from build123d import *

# Parameters (mm, degrees)
SKETCH1_W               = 359.9
SKETCH1_H               = 87.2
BOSS_EXTRUDE1_DEPTH     = 1.6256
SKETCH2_W               = 359.9
SKETCH2_H               = 87.2
SKETCH2_W_2             = 356.6488
SKETCH2_H_2             = 83.9488
BOSS_EXTRUDE2_DEPTH     = 69.85
SKETCH3_W               = 416.6488
SKETCH3_H               = 138
SKETCH3_W_2             = 356.6488
SKETCH3_H_2             = 83.9488
BOSS_EXTRUDE3_DEPTH     = 1.6256
FILLET1_R               = 1.905
SKETCH6_W               = 371.0088
SKETCH6_H               = 92.8388
BOSS_EXTRUDE4_DEPTH     = 3.175
SKETCH8_R               = 7.62
CUT_EXTRUDE2_DEPTH      = 402.075797246
CUT_EXTRUDE4_DEPTH      = 232.308973187
CUT_EXTRUDE4_DEPTH_BACK = 232.308973187
SKETCH17_W              = 28.095
SKETCH17_H              = 54
CUT_EXTRUDE5_DEPTH      = 232.308973187
CUT_EXTRUDE5_DEPTH_BACK = 232.308973187
SKETCH18_R              = 3.325


with BuildPart() as part:
    # Sketch1 → Boss-Extrude1 (new body)
    with BuildSketch(Plane(origin=(0, 0, 0), x_dir=(1, 0, 0), z_dir=(0, 1, 0))):
        Rectangle(SKETCH1_W, SKETCH1_H)
    extrude(amount=BOSS_EXTRUDE1_DEPTH)

    # Sketch2 → Boss-Extrude2 (add)
    with BuildSketch(Plane(origin=(0, 1.6256, 0), x_dir=(1, 0, 0), z_dir=(0, 1, 0))):
        Rectangle(SKETCH2_W, SKETCH2_H)
        Rectangle(SKETCH2_W_2, SKETCH2_H_2, mode=Mode.SUBTRACT)
    extrude(amount=BOSS_EXTRUDE2_DEPTH)

    # Sketch3 → Boss-Extrude3 (add)
    with BuildSketch(Plane(origin=(0, 71.4756, 0), x_dir=(1, 0, 0), z_dir=(0, 1, 0))):
        Rectangle(SKETCH3_W, SKETCH3_H)
        Rectangle(SKETCH3_W_2, SKETCH3_H_2, mode=Mode.SUBTRACT)
    extrude(amount=BOSS_EXTRUDE3_DEPTH)

    # Fillet1
    fillet1_edges = [part.edges().sort_by_distance(p)[0] for p in [
        (0, 71.4756, -43.6),
        (-179.95, 71.4756, 0),
        (0, 71.4756, 43.6),
        (179.95, 71.4756, 0),
        (-178.3244, 73.1012, 0),
        (0, 73.1012, 41.9744),
        (178.3244, 73.1012, 0),
        (0, 73.1012, -41.9744),
    ]]
    fillet(fillet1_edges, radius=FILLET1_R)

    # Sketch6 → Boss-Extrude4 (add)
    with BuildSketch(Plane(origin=(0, 73.1012, 0), x_dir=(1, 0, 0), z_dir=(0, 1, 0))):
        Polygon((188.2394, -49.5944), (-188.2394, -49.5944), (-191.4144, -49.5944), (-191.4144, 49.5944), (-188.2394, 49.5944), (188.2394, 49.5944), (191.4144, 49.5944), (191.4144, -49.5944), align=None)
        with Locations((-2.735, 0)):
            Rectangle(SKETCH6_W, SKETCH6_H, mode=Mode.SUBTRACT)
    extrude(amount=-BOSS_EXTRUDE4_DEPTH)

    # Sketch8 → Cut-Extrude2 (cut, through all)
    with BuildSketch(Plane(origin=(179.95, 0, 0), x_dir=(0, 0, -1), z_dir=(1, 0, 0))):
        with Locations((0, 12.7)):
            Circle(SKETCH8_R)
    extrude(amount=-CUT_EXTRUDE2_DEPTH, mode=Mode.SUBTRACT)

    # Sketch17 → Cut-Extrude4 (cut, two sides: drawn at the far end of the back side and taken through both)
    with BuildSketch(Plane(origin=(0, 73.1012, 0), x_dir=(1, 0, 0), z_dir=(0, 1, 0)).offset(-CUT_EXTRUDE4_DEPTH_BACK)):
        with Locations((194.2769, 0)):
            Rectangle(SKETCH17_W, SKETCH17_H)
    extrude(amount=CUT_EXTRUDE4_DEPTH + CUT_EXTRUDE4_DEPTH_BACK, mode=Mode.SUBTRACT)

    # Sketch18 → Cut-Extrude5 (cut, two sides: drawn at the far end of the back side and taken through both)
    with BuildSketch(Plane(origin=(0, 73.1012, 0), x_dir=(1, 0, 0), z_dir=(0, 1, 0)).offset(-CUT_EXTRUDE5_DEPTH_BACK)):
        with Locations(Location((203.37295269, 41.64816795, 0), (0, 0, 270))):
            Circle(SKETCH18_R)
        with Locations(Location((203.37295269, -41.64816795, 0), (0, 0, 90))):
            Circle(SKETCH18_R)
        with Locations(Location((129.76878637, 57.22406113, 0), (0, 0, 270))):
            Circle(SKETCH18_R)
        with Locations(Location((-50.23121363, 57.22406113, 0), (0, 0, 270))):
            Circle(SKETCH18_R)
        with Locations(Location((39.76878637, 57.22406113, 0), (0, 0, 270))):
            Circle(SKETCH18_R)
        with Locations(Location((-140.23121363, 57.22406113, 0), (0, 0, 270))):
            Circle(SKETCH18_R)
        with Locations(Location((129.76878637, -57.22406113, 0), (0, 0, 90))):
            Circle(SKETCH18_R)
        with Locations(Location((39.76878637, -57.22406113, 0), (0, 0, 90))):
            Circle(SKETCH18_R)
        with Locations(Location((-50.23121363, -57.22406113, 0), (0, 0, 90))):
            Circle(SKETCH18_R)
        with Locations(Location((-140.23121363, -57.22406113, 0), (0, 0, 90))):
            Circle(SKETCH18_R)
    extrude(amount=CUT_EXTRUDE5_DEPTH + CUT_EXTRUDE5_DEPTH_BACK, mode=Mode.SUBTRACT)


solid = part.part
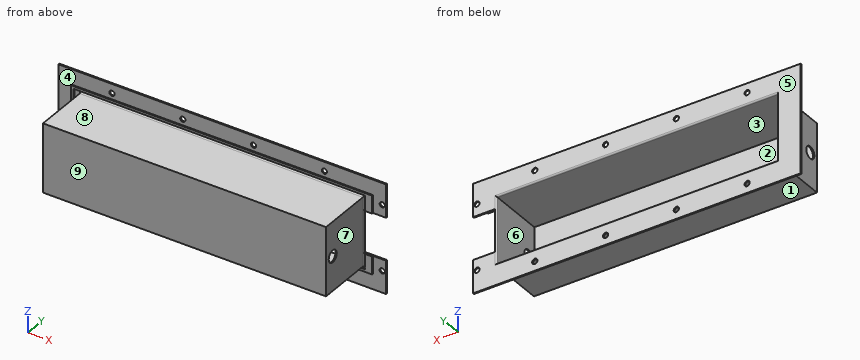
Can you work these out from the model? Positions are in its coordinate system, mm. Face numbers are marked on the shaded views. A direction names the side the tool comes from. Give positions to 0.01 mm unless a question says otherwise; leave off trailing zeros. Order: outer loops, then holes, each group sorted by start corner. A loop starts at its lowest first (then second) coordinate and runs counter-clockwise, first axis right, second up. Notation, with made-up numbers: M 58,18.5 L 67,18.5 A26 ccw 67,39.5 Z; hole C 31.25,68.25 d5. An arc over 180 degrees is marked long. Use a Markdown table: item, result. Add a question column.
Item 1: Suppose I cut it at B-B (y = 12.7). List the corners of the cut face in (x, z) for me, then the cut area to 3 significant figures.
Item 2: For the marked faces 5, 6, 7, 8 and 9, which set-ups out of +Z, -Z, +X, -X, +Y, -Y let a thin tool reach every point of the face, with its end or its side?
Item 3: Suppose I cut it at A-A (z = 0). List the corners of the cut face in (x, y) for me (3 decimals).
Item 4: We'd pull the mould along Z, two halves only. Please class the marked faces 1, 2, 3 and 4: +Z half, -Z half, draft (parallel to the pull), parting line (faces both ways), or undercut.
Item 5: Suppose I cut it at C-C (y = 52.5). List the corners of the cut face in (x, z) for me, then the cut area to 3 significant figures.
Item 6: If I drill on L1, parallel to Z at x = 88, y = 53.5; L2, parallel to X at y = 38, z = 18; L3, parallel to Z at x = -179, y = 12, over which ranges is the centre line in solid material (lowest first)? Write a range as [from, to].
Item 7: Suppose I cut it at D-D (x = -58). List the corners of the cut face in (y, z) for me (3 decimals).
Item 8: Will these pins go through, and if not, where does the flat tip stop? pin 1 (0.5 mm diameter, centred on y = 70.5, z = 38.5, fed in from -X); pin 2 (8 mm diameter, centred on y = 54.5, z = 31.5, fed in from -X); pin 3 (7.5 mm diameter, centred on x = -50.23, z = -57.22, fed in from -Y).
Answer sheet:
| question | item | result |
|---|---|---|
| 1 | outline | M -179.95,-43.6 L 179.95,-43.6 L 179.95,-7.62 L 178.32,-7.62 L 178.32,-41.97 L -178.32,-41.97 L -178.32,-7.62 L -179.95,-7.62 Z; M -179.95,7.62 L -178.32,7.62 L -178.32,41.97 L 178.32,41.97 L 178.32,7.62 L 179.95,7.62 L 179.95,43.6 L -179.95,43.6 Z |
| 1 | area | 1,390 mm² |
| 2 | face 5 | +Z, -Z, +X, -X, +Y |
| 2 | face 6 | +Y |
| 2 | face 7 | +Z, -Z, +X, -Y |
| 2 | face 8 | +Z, +X, -X, -Y |
| 2 | face 9 | +Z, -Z, +X, -X, -Y |
| 3 | outline | M -208.324,71.476 L -191.414,71.476 L -191.414,69.926 L -188.239,69.926 L -188.239,71.476 L -181.855,71.476 A1.905 cw -179.95,69.571 L -179.95,20.32 L -178.324,20.32 L -178.324,71.196 A1.905 ccw -180.229,73.101 L -208.324,73.101 Z; M -179.95,0 L 179.95,0 L 179.95,5.08 L 178.324,5.08 L 178.324,1.626 L -178.324,1.626 L -178.324,5.08 L -179.95,5.08 Z; M 178.324,20.32 L 179.95,20.32 L 179.95,69.571 A1.905 cw 180.229,70.564 L 180.229,73.101 A1.905 ccw 178.324,71.196 Z |
| 4 | face 1 | -Z half |
| 4 | face 2 | undercut |
| 4 | face 3 | undercut |
| 4 | face 4 | draft |
| 5 | outline | M -179.95,-43.6 L 179.95,-43.6 L 179.95,43.6 L -179.95,43.6 Z; hole M -178.32,-41.97 L 178.32,-41.97 L 178.32,41.97 L -178.32,41.97 Z |
| 5 | area | 1,440 mm² |
| 6 | L1 | z = [-43.6, -41.97], [41.97, 43.6] |
| 6 | L2 | x = [-179.95, -178.32], [178.32, 179.95] |
| 6 | L3 | z = [-43.6, -7.59], [7.59, 43.6] |
| 7 | outline | M 0,-43.6 L 69.571,-43.6 A1.905 cw 71.476,-45.505 L 71.476,-46.419 L 69.926,-46.419 L 69.926,-49.594 L 71.476,-49.594 L 71.476,-69 L 73.101,-69 L 73.101,-43.879 A1.905 ccw 71.196,-41.974 L 1.626,-41.974 L 1.626,41.974 L 71.196,41.974 A1.905 ccw 73.101,43.879 L 73.101,69 L 71.476,69 L 71.476,49.594 L 69.926,49.594 L 69.926,46.419 L 71.476,46.419 L 71.476,45.505 A1.905 cw 69.571,43.6 L 0,43.6 Z |
| 8 | pin 1 | stops at x = -191.41 |
| 8 | pin 2 | stops at x = -179.95 |
| 8 | pin 3 | stops at y = 71.48 |
